```python
from build123d import *

# Parameters (mm, degrees)
SKETCH_1_R      = 1.448445572
SKETCH_1_R_2    = 1.5
EXTRUDE_1_DEPTH = 3
EXTRUDE_2_DEPTH = 3
SKETCH_5_W      = 10
SKETCH_5_H      = 30
EXTRUDE_3_DEPTH = 3


with BuildPart() as part:
    # 草图1 → 凸台-拉伸1 (new body)
    with BuildSketch(Plane(origin=(0, 0, 0), x_dir=(1, 0, 0), z_dir=(0, 1, 0))):
        Polygon((0, 0), (-35, 0), (-35, -30), (-45, -30), (-45, 20), (45, 20), (45, -30), (35, -30), (35, 0), align=None)
        with Locations(Location((-42, -26, 0), (0, 0, 270))):
            Circle(SKETCH_1_R, mode=Mode.SUBTRACT)
        with Locations(Location((-42, 16, 0), (0, 0, 270))):
            Circle(SKETCH_1_R_2, mode=Mode.SUBTRACT)
        with Locations(Location((42, -26, 0), (0, 0, 90))):
            Circle(SKETCH_1_R, mode=Mode.SUBTRACT)
        with Locations(Location((42, 16, 0), (0, 0, 90))):
            Circle(SKETCH_1_R_2, mode=Mode.SUBTRACT)
    extrude(amount=EXTRUDE_1_DEPTH)

    # 草图2 → 凸台-拉伸2 (add)
    with BuildSketch(Plane(origin=(-35, 0, 0), x_dir=(0, 0, -1), z_dir=(1, 0, 0))):
        with BuildLine():
            Line((-9.320508076, 33), (-60.282676081, 121.269064248))
            ThreePointArc((-60.282676081, 121.269064248), (-60.782178193, 125.063159474), (-58.452549062, 128.099191267))
            Line((-58.452549062, 128.099191267), (-58.1128031, 128.29534369))
            ThreePointArc((-58.1128031, 128.29534369), (-54.318707874, 128.794845803), (-51.282676081, 126.465216671))
            Line((-51.282676081, 126.465216671), (20, 3))
            Line((20, 3), (8, 3))
            Line((8, 3), (-26.641016151, 3))
            ThreePointArc((-26.641016151, 3), (-9.320508076, 13), (-9.320508076, 33))
        make_face()
        with BuildLine():
            Line((-53.673261241, 122.605831628), (9.977098662, 12.360174356))
            ThreePointArc((9.977098662, 12.360174356), (9.428060557, 10.31113625), (7.379022451, 10.860174356))
            Line((7.379022451, 10.860174356), (-56.271337452, 121.105831628))
            ThreePointArc((-56.271337452, 121.105831628), (-55.722299346, 123.154869734), (-53.673261241, 122.605831628))
        make_face(mode=Mode.SUBTRACT)
    extrude_2 = extrude(amount=-EXTRUDE_2_DEPTH)

    # 镜向1: 凸台-拉伸2 across plane
    add(extrude_2.mirror(Plane(origin=(0, 0, 0), x_dir=(0, 0, 1), z_dir=(1, 0, 0))))

    # 草图5 → 凸台-拉伸3 (add)
    with BuildSketch(Plane.XZ):
        with Locations((-30, 15)):
            Rectangle(SKETCH_5_W, SKETCH_5_H)
        with Locations((30, 15)):
            Rectangle(SKETCH_5_W, SKETCH_5_H)
    extrude(amount=-EXTRUDE_3_DEPTH)


solid = part.part
```
Geometry check sheet. Reference: the model listing, model coordinates, mm. A direction names the side the tool comes from. Round coordinates to 2 decimals unless told otherwise and drop trailing zeros. Order: outer loops, then holes, each group sorted by start corner. A loop starts at its lowest first (then second) coordinate and runs counter-clockwise, first axis right, second up. Notation, with made-up numbers: (35.25, 0.25) - (42.25, 0.25) arc R23 ccw to (42.25, 10.25) - close; hole circle Ø7 at (42.25, -14). An arc over 180 degrees is marked (long way). Use a Markdown table: item, result. Add a question column.
1) Thickness scan on line 1 along Z through (x, y) = (42, 0.95); line 2 along X through (y, z) = (1.6, -16); line 3 along X through (y, z) = (2.15, 26). Record the ranges inside material, lowest first.
2) Mould release check, pull along Y, two halves, no side actions. Record for faces 5 (the flat face through (-36.48, 65.6, 16.14)), 6 (the cylindrical face through (43.464, 1.479, -15.675)), 7 (the cylindrical face through (36.479, 12.747, 9.469)): released by +Y, released by -Y, zero draft, split by the parting line, or undercut.
3) Section check B-B (z = 22.5). Count the separate pieces of the cut face and the enclosed holes in it, then the cut area to 3 significant figures.
4) Section check C-C (z = -16). Record the cut outline in (x, y).
5) Section check A-A (x = 42). Record the cut outline in (y, z).
6) Gauge pin test, flat ends, axial feed: P1, Ø0.9, axis at x = -35.5, y = 2, coming from the +Z side; P2, Ø3, axis at x = -29.5, z = 21, coming from the +Y side; P3, Ø6, axis at y = 24, z = 11.5, coming from the +X side; P4, Ø1.5, axis at y = 21, z = -7.5, coming from the -X side. Record the tip position at first contact, or that the pin passes through.
7) Set-up check for faces 1 (the flat face through (36.48, 68.25, 22.29)), 2 (the flat face through (35, 52, 17)), 3 (the flat face through (36.479, 76.517, 34.445)), 4 (the flat face through (25, 1, 15)): record each of +Z, -Z, +X, -X, +Y, -Y from which the full face is reachable in a straight line by a thin tool's end or side.
8) Section check D-D (y = 14.5). Record the cut outline in (x, z).
Established:
| question | item | result |
|---|---|---|
| 1 | line 1 | -20 to -17.5, -14.5 to 24.55, 27.45 to 30 |
| 1 | line 2 | -45 to -43.5, -40.5 to 40.5, 43.5 to 45 |
| 1 | line 3 | -45 to -43.45, -40.55 to -25, 25 to 40.55, 43.45 to 45 |
| 2 | face 5 | released by +Y |
| 2 | face 6 | zero draft |
| 2 | face 7 | undercut |
| 3 | separate pieces | 6 |
| 3 | enclosed holes | 0 |
| 3 | area | 211 mm2 |
| 4 | outline | (-45, 0) - (-43.5, 0) - (-43.5, 3) - (-45, 3) - close; (-40.5, 0) - (40.5, 0) - (40.5, 3) - (38, 3) - (38, 9.93) - (35, 9.93) - (35, 3) - (-35, 3) - (-35, 9.93) - (-38, 9.93) - (-38, 3) - (-40.5, 3) - close; (43.5, 0) - (45, 0) - (45, 3) - (43.5, 3) - close |
| 5 | outline | (0, -20) - (3, -20) - (3, -17.5) - (0, -17.5) - close; (0, -14.5) - (3, -14.5) - (3, 24.55) - (0, 24.55) - close; (0, 27.45) - (3, 27.45) - (3, 30) - (0, 30) - close |
| 6 | P1 | z = 30 |
| 6 | P2 | y = 3 |
| 6 | P3 | through |
| 6 | P4 | x = -38 |
| 7 | face 1 | +X, -X |
| 7 | face 2 | +Z, -Z, +Y |
| 7 | face 3 | +Z, +X, -X |
| 7 | face 4 | +Z, +Y, -Y |
| 8 | outline | (-38, -13.36) - (-35, -13.36) - (-35, -8.74) - (-38, -8.74) - close; (-38, -5.28) - (-35, -5.28) - (-35, 8.54) - (-38, 8.54) - close; (35, -13.36) - (38, -13.36) - (38, -8.74) - (35, -8.74) - close; (35, -5.28) - (38, -5.28) - (38, 8.54) - (35, 8.54) - close |
